from build123d import *

# Parameters (mm, degrees)
SCHIZZO1_R                   = 6
ESTRUSIONE_ESTRUSIONE1_DEPTH = 200
SCHIZZO2_W                   = 10
SCHIZZO2_H                   = 6
ESTRUSIONE_ESTRUSIONE2_DEPTH = 10
SCHIZZO6_W                   = 2.625434249
SCHIZZO6_H                   = 12.677495408
TAGLIO_ESTRUSIONE1_DEPTH     = 10
RACCORDO2_R                  = 1
RACCORDO3_R                  = 1


with BuildPart() as part:
    # Schizzo1 → Estrusione-Estrusione1 (new body)
    with BuildSketch(Plane.XY):
        with Locations(Location((0, 0, 0), (0, 0, 180))):
            Circle(SCHIZZO1_R)
    extrude(amount=ESTRUSIONE_ESTRUSIONE1_DEPTH)

    # Schizzo2 → Estrusione-Estrusione2 (add)
    with BuildSketch(Plane.XY.offset(200)):
        Rectangle(SCHIZZO2_W, SCHIZZO2_H)
    extrude(amount=ESTRUSIONE_ESTRUSIONE2_DEPTH)

    # Schizzo6 → Taglio-Estrusione1 (cut)
    with BuildSketch(Plane(origin=(0, 0, 0), x_dir=(-1, 0, 0), z_dir=(0, 0, -1))):
        with Locations((4.687282876, 0.338747704)):
            Rectangle(SCHIZZO6_W, SCHIZZO6_H)
        with Locations((-4.687282876, 0.338747704)):
            Rectangle(SCHIZZO6_W, SCHIZZO6_H)
    extrude(amount=-TAGLIO_ESTRUSIONE1_DEPTH, mode=Mode.SUBTRACT)

    # Raccordo2
    raccordo2_edges = [part.edges().sort_by_distance(p)[0] for p in [
        (3.374565751, 0, 10),
    ]]
    fillet(raccordo2_edges, radius=RACCORDO2_R)

    # Raccordo3
    raccordo3_edges = [part.edges().sort_by_distance(p)[0] for p in [
        (-3.374565751, 0, 10),
    ]]
    fillet(raccordo3_edges, radius=RACCORDO3_R)


solid = part.part
The model under review builds one solid part; all positions refer to its coordinate system, in mm. A direction names the side the tool comes from. Round coordinates to 2 decimals unless told otherwise and drop trailing zeros. Write each loop counter-clockwise with the first axis right and the second up, starting at its lowest first coordinate (ties: lowest second). Pieces come first, ordered by that corner, then holes. Notation, with made-up numbers: (-32.5, -21) -> (6.5, -21) arc R26 ccw to (6.5, -6) -> close; hole circle Ø10 at (-28.5, -27.5). An arc over 180 degrees is marked (long way). Answer as a JSON object with one key per item and string values.
1. We need section A-A on y = 0. State the section outline as (x, z) points.
Results found:
{"outline": "(-6, 10) -> (-4.37, 10) arc R1 cw to (-3.37, 9) -> (-3.37, 0) -> (3.37, 0) -> (3.37, 9) arc R1 cw to (4.37, 10) -> (6, 10) -> (6, 200) -> (5, 200) -> (5, 210) -> (-5, 210) -> (-5, 200) -> (-6, 200) -> close"}
2. Machinability: for faces 1 (the face through (0, 3, 205)), 2 (the face through (5, 0, 205)), 3 (the face through (-3.375, 0, 4)), which of the approach directions +Z, -Z, +X, -X, +Y, -Y give a long, thin tool a straight path to every point of the face, cutting with its end or side? Answer none if there is none.
Results found:
{"face 1": "+Z, +X, -X, +Y", "face 2": "+Z, +X, +Y, -Y", "face 3": "-Z, -X, +Y, -Y"}
3. We need section C-C on z = 24.5. State the section outline as (x, y) points.
Results found:
{"outline": "circle Ø12 at (0, 0)"}
4. The part is to be moulded in two halves that separate along Z. For faces 4 (the face through (0, 0, 0)), 5 (the face through (3.375, 0, 4)), 6 (the face through (0, 0, 210)), say which applies: pulls with the +Z half, pulls with the -Z half, needs draft (parallel to the pull), parting line crosses it, or undercut.
Results found:
{"face 4": "pulls with the -Z half", "face 5": "needs draft", "face 6": "pulls with the +Z half"}
5. We need section B-B on x = 0. State the section outline as (y, z) points, and give its area (3 significant figures).
Results found:
{"outline": "(-6, 0) -> (6, 0) -> (6, 200) -> (3, 200) -> (3, 210) -> (-3, 210) -> (-3, 200) -> (-6, 200) -> close", "area": "2,460 mm^2"}
6. To check wall thickness, follow line 1 along Y through (x, z) = (-2, 201.5); line 2 along Z through (x, y) = (-0.5, -3.25); line 3 along Y through (x, z) = (-2.5, 190.5). State the ranges of each line that lie inside material, in increasing order.
Results found:
{"line 1": "y = -3 to 3", "line 2": "z = 0 to 200", "line 3": "y = -5.45 to 5.45"}
7. Clearance check with flat-ended pins moving along their axes: pin 1 (6.5 mm diameter, centred on y = -0.5, z = 204, fed in from +X); pin 2 (3 mm diameter, centred on x = -4.5, z = 187.5, fed in from +Y); pin 3 (2.5 mm diameter, centred on y = 1.5, z = 5.5, fed in from -X). State where each tip first meets the part, or that it passes through.
Results found:
{"pin 1": "stops at x = 5", "pin 2": "stops at y = 5.2", "pin 3": "stops at x = -3.37"}
